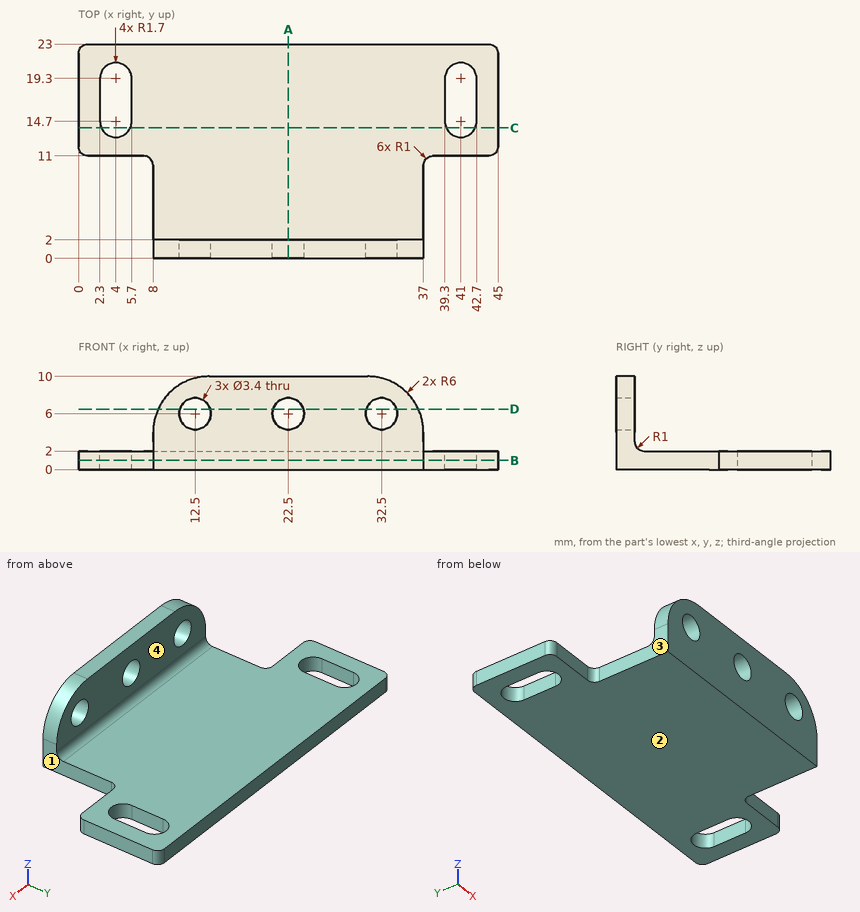
Study the drawing (mm; zero at the part's minimum x, y, z) and answer. A direction names the side the tool comes from. Round coordinates to 2 decimals unless told otherwise and drop trailing zeros. Loops run counter-clockwise (first coordinate to the right, second up) from the corner with the lowest first, then second, coordinate; pieces in that order, holes last. Notation, with made-up numbers: (49.5, -21) -> (67.5, -21) arc R25 cw to (67.5, 0) -> close; hole circle Ø7 at (73, -29.5). An arc over 180 degrees is marked (long way). Use one line per item in the form item = value.
1. The part is cut by section B-B on z = 1. Determine the outline of the cut face in (x, y), and give its area (3 significant figures).
Answer key:
outline = (0, 12) arc R1 ccw to (1, 11) -> (7, 11) arc R1 cw to (8, 10) -> (8, 0) -> (37, 0) -> (37, 10) arc R1 cw to (38, 11) -> (44, 11) arc R1 ccw to (45, 12) -> (45, 22) arc R1 ccw to (44, 23) -> (1, 23) arc R1 ccw to (0, 22) -> close; hole (2.3, 14.7) arc R1.7 ccw to (5.7, 14.7) -> (5.7, 19.3) arc R1.7 ccw to (2.3, 19.3) -> close; hole (39.3, 14.7) arc R1.7 ccw to (42.7, 14.7) -> (42.7, 19.3) arc R1.7 ccw to (39.3, 19.3) -> close
area = 809 mm²
2. Flat-ended cylindrical pins translate along their axes: pin 1 Ø2 at (y, z) = (7.5, 1.5) entering from +X; pin 2 Ø2 at (x, z) = (27.5, 8) entering from +Y; pin 3 Ø2 at (x, z) = (5, 1) entering from -Y. Find the tip coordinate at first contact, or state that the pin passes through.
Answer key:
pin_1 = 37
pin_2 = 2
pin_3 = 11
3. Find the intervals of material crossed by probe 1 along X at (y, z) = (0.7, 6); probe 2 along Z at (x, y) = (22, 8); probe 3 along Z at (x, y) = (22.5, 0.8), in increasing order. Write a range as [from, to].
Answer key:
probe_1 = [8.34, 10.8], [14.2, 20.8], [24.2, 30.8], [34.2, 36.66]
probe_2 = [0, 2]
probe_3 = [0, 4.3], [7.7, 10]
4. The part is cut by section C-C on y = 14. Determine the outline of the cut face in (x, z), and give its area (3 significant figures).
Answer key:
outline = (0, 0) -> (2.45, 0) -> (2.45, 2) -> (0, 2) -> close; (5.55, 0) -> (39.45, 0) -> (39.45, 2) -> (5.55, 2) -> close; (42.55, 0) -> (45, 0) -> (45, 2) -> (42.55, 2) -> close
area = 77.6 mm²
5. The part is cut by section D-D on z = 6.5. Determine the outline of the cut face in (x, y).
Answer key:
outline = (8.55, 0) -> (10.88, 0) -> (10.88, 2) -> (8.55, 2) -> close; (14.12, 0) -> (20.88, 0) -> (20.88, 2) -> (14.12, 2) -> close; (24.12, 0) -> (30.88, 0) -> (30.88, 2) -> (24.12, 2) -> close; (34.12, 0) -> (36.45, 0) -> (36.45, 2) -> (34.12, 2) -> close
6. The part is cut by section A-A on x = 22.5. Determine the outline of the cut face in (y, z).
Answer key:
outline = (0, 0) -> (23, 0) -> (23, 2) -> (3, 2) arc R1 cw to (2, 3) -> (2, 4.3) -> (0, 4.3) -> close; (0, 7.7) -> (2, 7.7) -> (2, 10) -> (0, 10) -> close
7. A tool of negligible diameter and unlimited length cuts with its end or side. For the marked faces 1, 2, 3 and 4, from which of +Z, -Z, +X, -X, +Y, -Y can it reach the whole face along a straight path? Write none if from no direction.
Answer key:
face_1 = +Z, -Z, +X, -Y
face_2 = -Z, +X, -X, +Y, -Y
face_3 = +Z, -Z, -X, -Y
face_4 = +Z, +X, -X, +Y
